from build123d import *

# Parameters (mm, degrees)
F1_DEPTH = 63.5
F0_W     = 17.9729990546
F0_H     = 19.05
F2_DEPTH = 25.4
F3_DEPTH = 7.9375


with BuildPart() as f1:
    # F0 (on Front) → F1 (new body, symmetric)
    with BuildSketch(Plane.XZ):
        Polygon((22.225, 9.525), (-41.275, 9.525), (-41.275, -9.525), (41.275, -9.525), (41.275, 9.525), align=None)
    extrude(amount=F1_DEPTH, both=True)

    # F0 (on Front) → F2 (join, symmetric)
    with BuildSketch(Plane.XZ):
        with BuildLine():
            Line((22.225, 27.0002), (22.225, 9.525))
            Line((22.225, 9.525), (41.275, 9.525))
            Line((41.275, 9.525), (41.275, 27.0002))
            ThreePointArc((41.275, 27.0002), (45.9246798487, 38.2255201513), (57.15, 42.8752))
            Line((57.15, 42.8752), (60.325, 42.8752))
            Line((60.325, 42.8752), (60.325, 61.9252))
            Line((60.325, 61.9252), (57.15, 61.9252))
            add(Edge.make_bspline(
                [(54.2615577604, 61.8055519797), (55.2288783664, 61.8546366141), (56.1919158349, 61.8945538675), (57.15, 61.9252)],
                knots=[109.0649355022, 109.0649355022, 109.0649355022, 109.0649355022, 111.5045361635, 111.5045361635, 111.5045361635, 111.5045361635], degree=3))
            ThreePointArc((54.2615577604, 61.8055519797), (31.4533614045, 50.6526499765), (22.225, 27.0002))
        make_face()
        with Locations((69.3114995273, 52.4002)):
            Rectangle(F0_W, F0_H)
    extrude(amount=F2_DEPTH, both=True)

    # F0 (on Front) → F3 (join, symmetric)
    with BuildSketch(Plane.XZ):
        with BuildLine():
            add(Edge.make_bspline(
                [(-41.275, 9.525), (-40.7890449991, 39.0945706255), (11.0164639317, 59.6111713264), (54.2615577604, 61.8055519797)],
                knots=[0, 0, 0, 0, 109.0649355022, 109.0649355022, 109.0649355022, 109.0649355022], degree=3))
            Line((-41.275, 9.525), (22.225, 9.525))
            Line((22.225, 9.525), (22.225, 27.0002))
            ThreePointArc((22.225, 27.0002), (31.4533614045, 50.6526499765), (54.2615577604, 61.8055519797))
        make_face()
    extrude(amount=F3_DEPTH, both=True)

    # F0 (on Front) → F4 (revolve)
    with BuildSketch(Plane.XZ):
        Polygon((60.325, 66.675), (60.325, 61.9252), (78.2979990546, 61.9252), (78.2979990546, 42.8752), (60.325, 42.8752), (60.325, 38.1), (111.125, 38.1), (111.125, 66.675), align=None)
    revolve(axis=Axis((60.325, 0, 52.3875), (0, 0, 1)))


solid = f1.part
The listing builds one solid part. Answer for the finished solid, in the listing's coordinates (mm). A direction names the side the tool comes from. Round coordinates to 2 decimals unless told otherwise and drop trailing zeros. Order: outer loops, then holes, each group sorted by start corner. A loop starts at its lowest first (then second) coordinate and runs counter-clockwise, first axis right, second up. Notation, with made-up numbers: M 66,62.5 L 76,62.5 A26 ccw 76,97.5 Z; hole C 62,47 d3. An arc over 180 degrees is marked long. Answer in a Markdown table with one row per item. Add a question column.
1) Determine the mould class of faces 1 (the face through (22.225, 17, 18)), 2 (the face through (-1, -1, -9.525)), 3 (the face through (-8, -7.938, 27)), 4 (the face through (-1, 63.5, 0)) for opening direction Z: pulls with the +Z half, pulls with the -Z half, needs draft (parallel to the pull), parting line crosses it, or undercut.
2) The part is cut by section B-B on z = 7. Determine the outline of the cut face in (x, y) (3 decimals), plus the area to 3 significant figures.
3) The part is cut by section D-D on y = -46. Determine the outline of the cut face in (x, z) (1 decimal).
4) Consider line 1 along Z through (x, y) = (34, -29) (3 decimals); line 2 along Z through (x, y) = (10, 47) (3 decimals); line 3 along X through (y, z) = (-45.5, -4.5) (3 decimals). Determine where each line is inside the solid, lowest interval first. Write a range as from..to.
5) The part is cut by section A-A on y = 36. Determine the outline of the cut face in (x, z) (3 decimals), plus the area to 3 significant figures.
6) Flat-ended cylindrical pins translate along their axes: pin 1 Ø8 at (x, z) = (26, 28.5) entering from -Y; pin 2 Ø12 at (x, z) = (34, 29) entering from +Y; pin 3 Ø2 at (x, z) = (4.5, 12.5) entering from -Y. Find the tip coordinate at first contact, or state that the pin passes through.
7) The part is cut by section C-C on y = 23. Determine the outline of the cut face in (x, z) (3 decimals), plus the area to 3 significant figures.
8) Which of the six approach directions +Z, -Z, +X, -X, +Y, -Y give full straight-line access (tool end or side, diameter ignored) to faces 5 (the face through (22.225, -17, 18)), 6 (the face through (41.275, -1, 4)), 7 (the face through (42.355, 0.351, 61.216))?
Findings below:
| question | item | result |
|---|---|---|
| 1 | face 1 | undercut |
| 1 | face 2 | pulls with the -Z half |
| 1 | face 3 | undercut |
| 1 | face 4 | needs draft |
| 2 | outline | M -41.275,-63.5 L 41.275,-63.5 L 41.275,63.5 L -41.275,63.5 Z |
| 2 | area | 10,500 mm² |
| 3 | outline | M -41.3,-9.5 L 41.3,-9.5 L 41.3,9.5 L -41.3,9.5 Z; M 38.8,38.1 L 81.9,38.1 L 81.9,66.7 L 38.8,66.7 Z |
| 4 | line 1 | z = -9.525..9.525, 38.1..66.675 |
| 4 | line 2 | z = -9.525..9.525 |
| 4 | line 3 | x = -41.275..41.275 |
| 5 | outline | M -41.275,-9.525 L 41.275,-9.525 L 41.275,9.525 L -41.275,9.525 Z; M 24.483,38.1 L 96.167,38.1 L 96.167,66.675 L 24.483,66.675 Z |
| 5 | area | 3,620 mm² |
| 6 | pin 1 | stops at y = -25.4 |
| 6 | pin 2 | stops at y = 25.4 |
| 6 | pin 3 | stops at y = -7.94 |
| 7 | outline | M -41.275,-9.525 L 41.275,-9.525 L 41.275,27 A15.875 cw 45.801,38.1 L 105.62,38.1 L 105.62,66.675 L 15.03,66.675 L 15.03,38.1 L 24.036,38.1 A34.925 ccw 22.225,27 L 22.225,9.525 L -41.275,9.525 Z |
| 7 | area | 4,710 mm² |
| 8 | face 5 | -X, -Y |
| 8 | face 6 | -Z, +X, +Y, -Y |
| 8 | face 7 | none |
